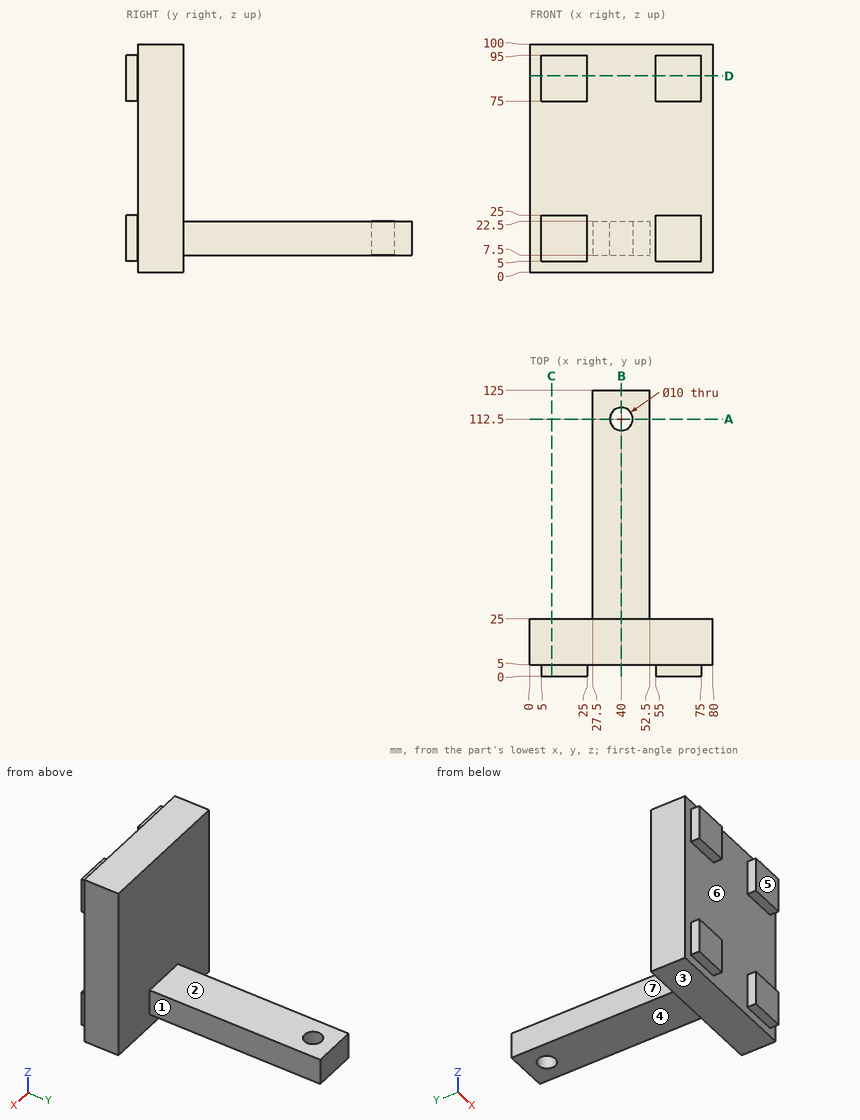
Study the drawing (mm; zero at the part's minimum x, y, z) and answer. A direction names the side the tool comes from. Give positions to 0.01 mm unless a question says otherwise; leave off trailing zeros. Write each loop counter-clockwise with the first axis right and the second up, starting at its lowest first coordinate (ties: lowest second). Pieces come first, ordered by that corner, then holes.
Item 1: Section B-B, the plane x = 40 is taken. Write down the section's boundary in (y, z).
Item 2: Flat-ended cylindrical pins translate along their axes: P1, Ø16.5, axis at y = 59.5, z = 11.5, coming from the -X side; P2, Ø5, axis at x = 15.5, z = 57.5, coming from the -Y side; P3, Ø1, axis at x = 12.5, z = 54, coming from the +Y side. Find the tip coordinate at first contact, or state that the pin passes through.
Item 3: Which of the six approach directions +Z, -Z, +X, -X, +Y, -Y give full straight-line access (tool end or side, diameter ignored) to the marked faces 1, 2, 3 and 4?
Item 4: Find the intervals of material crossed by line 1 along Y through (x, z) = (40, 19); line 2 along X through (y, z) = (112, 18); line 3 along Z through (x, y) = (42, 84.5), in increasing order.
Item 5: Section A-A, the plane y = 112.5 is taken. Write down the section's boundary in (x, z).
Item 6: Section C-C, the plane x = 9.5 is taken. Write down the section's boundary in (y, z).
Item 7: Determine the mould class of the marked faces 5, 6 and 7 for opening direction X: released by +X, released by -X, zero draft, split by the parting line, or undercut.
Item 8: Section D-D, the plane z = 86 is taken. Write down the section's boundary in (x, y).
Completed:
1. outline: (5, 0) - (25, 0) - (25, 7.5) - (107.5, 7.5) - (107.5, 22.5) - (25, 22.5) - (25, 100) - (5, 100) - close; (117.5, 7.5) - (125, 7.5) - (125, 22.5) - (117.5, 22.5) - close
2. P1: stops at x = 27.5
2. P2: stops at y = 5
2. P3: stops at y = 25
3. face 1: +Z, -Z, +X, +Y
3. face 2: +Z, +X, -X, +Y
3. face 3: -Z, +X, -X, +Y, -Y
3. face 4: -Z, +X, -X, +Y
4. line 1: y = 5 to 107.5, 117.5 to 125
4. line 2: x = 27.5 to 35.03, 44.97 to 52.5
4. line 3: z = 7.5 to 22.5
5. outline: (27.5, 7.5) - (35, 7.5) - (35, 22.5) - (27.5, 22.5) - close; (45, 7.5) - (52.5, 7.5) - (52.5, 22.5) - (45, 22.5) - close
6. outline: (0, 5) - (5, 5) - (5, 0) - (25, 0) - (25, 100) - (5, 100) - (5, 95) - (0, 95) - (0, 75) - (5, 75) - (5, 25) - (0, 25) - close
7. face 5: zero draft
7. face 6: undercut
7. face 7: released by -X
8. outline: (0, 5) - (5, 5) - (5, 0) - (25, 0) - (25, 5) - (55, 5) - (55, 0) - (75, 0) - (75, 5) - (80, 5) - (80, 25) - (0, 25) - close
